Could you check a few things on this model? Use its own coordinates, in mm. Coordinates: 2 decimals unless noted, no trailing zeros. Loops run counter-clockwise (first coordinate to the right, second up) from the corner with the lowest first, then second, coordinate; pieces in that order, holes last.
1) Imagine slicing it at B-B on x = 59.5. Please give me the cut outline in (y, z), plus the area to 3 significant figures.
2) Will these pins go through, and if not, where does the flat tip stop? P1, Ø12, axis at x = 107.5, y = -14, coming from the -Z side; P2, Ø12, axis at x = 76.5, y = -13.5, coming from the +Z side; P3, Ø1.6, axis at x = -5, z = 1, coming from the -Y side; P4, Ø1, axis at x = -2.5, z = 1.5, coming from the +Y side.
3) If I drill on line 1 along Z through (x, y) = (85, -15.75); line 2 along X through (y, z) = (-8.25, 5.7), over which ranges is the centre line in solid material (lowest first)?
4) Imagine slicing it at A-A on y = -2.75. Please give me the cut outline in (x, z), plus the area to 3 significant figures.
5) Thinking about a two-plate mould opening in Z: for faces 1 (the face through (147, -9, 4.2)), 2 (the face through (141.483, -9, 5)), 3 (the face through (147, -9, 6)), 4 (the face through (73, -9, 0)), which applies, released by +Z, released by -Z, zero draft, split by the parting line, or undercut?
```python
from build123d import *

# Parameters (mm, degrees)
SALIENTE_EXTRUIR1_DEPTH = 2
SALIENTE_EXTRUIR2_DEPTH = 10


with BuildPart() as part:
    # Croquis1 → Saliente-Extruir1 (new body)
    with BuildSketch(Plane.XY):
        Polygon((-8.516541248, 1.295896328), (1.483458752, 1.295896328), (1.483458752, 3.295896328), (151.483458752, 3.295896328), (151.483458752, -20.704103672), (1.483458752, -20.704103672), (1.483458752, -18.704103672), (-8.516541248, -18.704103672), align=None)
    extrude(amount=SALIENTE_EXTRUIR1_DEPTH)

    # Croquis3 → Saliente-Extruir2 (add)
    with BuildSketch(Plane(origin=(151.483458752, 0, 0), x_dir=(0, 0, -1), z_dir=(1, 0, 0))):
        Polygon((-2, 1.545896328), (-2, 3.295896328), (-6, 3.295896328), (-6, -20.704103672), (-2, -20.704103672), (-2, -18.954103672), (-4.2, -18.954103672), (-4.2, 1.545896328), align=None)
    extrude(amount=-SALIENTE_EXTRUIR2_DEPTH)


solid = part.part
```
Filled in:
1. outline: (-20.7, 0) - (3.3, 0) - (3.3, 2) - (-20.7, 2) - close
1. area: 48.0 mm2
2. P1: stops at z = 0
2. P2: stops at z = 2
2. P3: stops at y = -18.7
2. P4: stops at y = 1.3
3. line 1: z = 0 to 2
3. line 2: x = 141.48 to 151.48
4. outline: (-8.52, 0) - (151.48, 0) - (151.48, 2) - (-8.52, 2) - close; (141.48, 4.2) - (151.48, 4.2) - (151.48, 6) - (141.48, 6) - close
4. area: 338 mm2
5. face 1: undercut
5. face 2: zero draft
5. face 3: released by +Z
5. face 4: released by -Z
